Input: dimensioned drawing with shaded views. Units: mm. Origin: part minimum x, y, z. Give positions to 0.01 mm unless a question says otherwise; leave off trailing zeros. Write each loop counter-clockwise with the first axis right and the second up, starting at its lowest first coordinate (ties: lowest second). Pieces come first, ordered by that corner, then holes. Notation, with made-up numbers: M 71.5,-39.75 L 81.5,-39.75 A25 ccw 81.5,-21.75 Z; hole C 65.5,11.25 d5. An arc over 180 degrees is marked long. Answer as a JSON object with one key per item and string values.
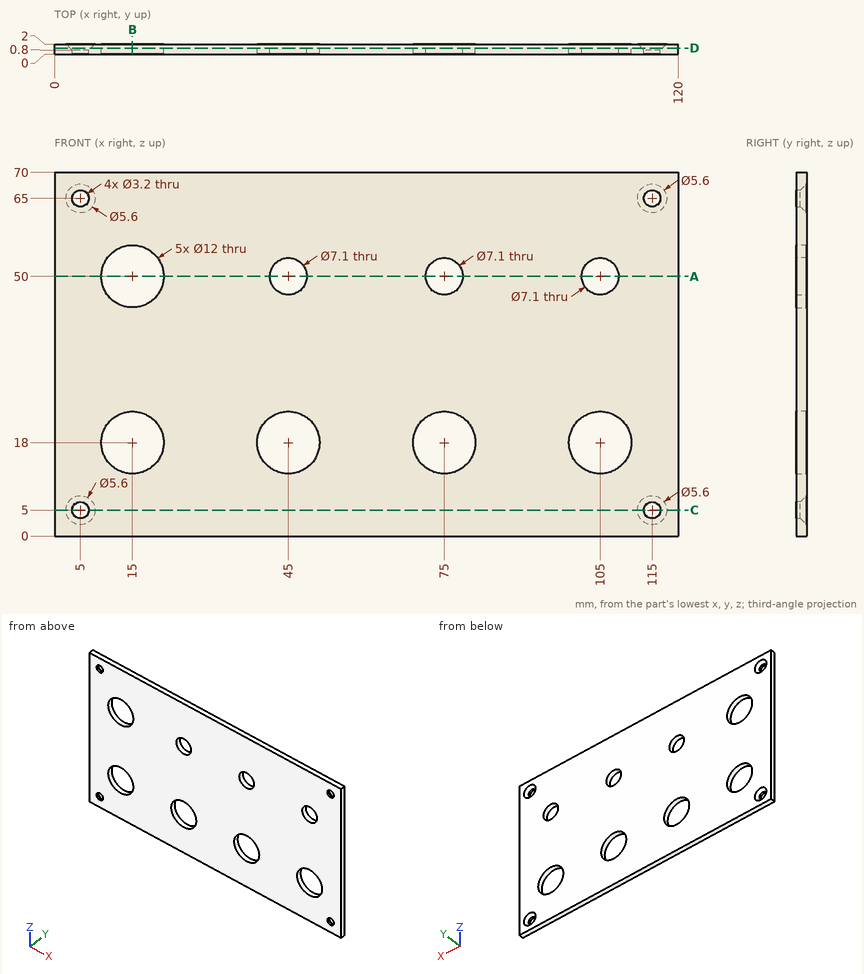
1) Contact query for a flat-ended pin moving along its axis: P1, Ø3.5, axis at x = 5, z = 65, coming from the +Y side. Output: stop coordinate, or through.
Geometry check:
{"P1": "stops at y = 0.95"}
2) Cut plane D-D on y = 1.2. Give the number of separate pieces and of enclosed holes in the cut face, and give its area (3 significant figures).
Geometry check:
{"separate pieces": "1", "enclosed holes": "12", "area": "7,670 mm2"}
3) Cut plane B-B on x = 15. Return loops of the section in (y, z).
Geometry check:
{"outline": "M 0,0 L 2,0 L 2,12 L 0,12 Z; M 0,24 L 2,24 L 2,44 L 0,44 Z; M 0,56 L 2,56 L 2,70 L 0,70 Z"}
4) Cut plane A-A on z = 50. Return loops of the section in (x, y), and give its area (3 significant figures).
Geometry check:
{"outline": "M 0,0 L 9,0 L 9,2 L 0,2 Z; M 21,0 L 41.45,0 L 41.45,2 L 21,2 Z; M 48.55,0 L 71.45,0 L 71.45,2 L 48.55,2 Z; M 78.55,0 L 101.45,0 L 101.45,2 L 78.55,2 Z; M 108.55,0 L 120,0 L 120,2 L 108.55,2 Z", "area": "173 mm2"}
5) Line query: line 1 (X direction, y = 0.6, z = 5); line 2 (X direction, y = 1.05, z = 18); line 3 (X direction, y = 0.35, z = 23). Output: solid intervals per line, ascending. Write a range as from..to.
Geometry check:
{"line 1": "x = 0..3.4, 6.6..113.4, 116.6..120", "line 2": "x = 0..9, 21..39, 51..69, 81..99, 111..120", "line 3": "x = 0..11.68, 18.32..41.68, 48.32..71.68, 78.32..101.68, 108.32..120"}
6) Cut plane C-C on z = 5. Return loops of the section in (x, y).
Geometry check:
{"outline": "M 0,0 L 3.4,0 L 3.4,0.8 L 2.2,2 L 0,2 Z; M 6.6,0 L 113.4,0 L 113.4,0.8 L 112.2,2 L 7.8,2 L 6.6,0.8 Z; M 116.6,0 L 120,0 L 120,2 L 117.8,2 L 116.6,0.8 Z"}
